Model file for the job. Use its own axes, mm. A direction names the side the tool comes from. Round coordinates to 2 decimals unless told otherwise and drop trailing zeros. Loops run counter-clockwise (first coordinate to the right, second up) from the corner with the lowest first, then second, coordinate; pieces in that order, holes last. Notation, with made-up numbers: M -4,5 L 11,5 A12 ccw 11,10 Z; hole C 28.5,-15.75 d1. An arc over 180 degrees is marked long. Answer in a Markdown table with one row per item.
Autodesk Inventor part; units mm, degrees
ref_plane "YZ Plane" through (0, 0, 0) normal (1, 0, 0) x (0, 1, 0)
ref_plane "XZ Plane" through (0, 0, 0) normal (0, 1, 0) x (-1, 0, 0)
ref_plane "XY Plane" through (0, 0, 0) normal (0, 0, 1) x (1, 0, 0)
sketch "Sketch1" plane through (0, 0, 0) normal (0, 0, 1) x (1, 0, 0)
  line L0 (0, 0) -> (-78.3, 0)
  line L1 (-78.3, 0) -> (-78.3, 100)
  line L2 (-78.3, 100) -> (0, 100)
  line L3 (0, 100) -> (0, 0)
  circle A0 centre (-11.5, 10) radius 1.5
  circle A1 centre (-11.5, 31.4) radius 1.5
  circle A2 centre (-14.5, 48.9) radius 1.5
  circle A3 centre (-27.5, 48.9) radius 1.5
  circle A4 centre (-70.8, 92.5) radius 1.5
  circle A5 centre (-70.8, 82.5) radius 1.5
  circle A6 centre (-70.8, 72.5) radius 1.5
  line L4 (0, 56.4) -> (-28.3, 56.4)
  line L5 (-28.3, 56.4) -> (-58.3, 86.4)
  line L6 (-58.3, 86.4) -> (-58.3, 100)
  line L7 (-30, 0) -> (-78.3, 48.3)
  dimension "d0" = 100
  dimension "d1" = 78.3
  dimension "d2" = 3
  dimension "d3" = 3
  dimension "d4" = 3
  dimension "d5" = 3
  dimension "d6" = 3
  dimension "d7" = 3
  dimension "d8" = 3
  dimension "d9" = 7.5
  dimension "d10" = 7.5
  dimension "d11" = 7.5
  dimension "d12" = 7.5
  dimension "d13" = 10
  dimension "d14" = 10
  dimension "d15" = 11.5
  dimension "d16" = 10
  dimension "d17" = 11.5
  dimension "d18" = 14.5
  dimension "d19" = 21.4
  dimension "d23" = 28.3
  dimension "d24" = 135
  dimension "d25" = 135
  dimension "d26" = 48.3
  dimension "d27" = 56.4
  dimension "d28" = 20
  dimension "d31" = 13
  dimension "d32" = 17.5
  dimension "d45" = 17.5
extrude "Extrusion1" add sketch "Sketch1" along normal blind 6 contours L0 L7 L1 L2 L6 L5 L4 L3
sketch "Sketch2" plane through (0, 0, 6) normal (0, 0, 1) x (1, 0, 0)
  line L0 (-30, 0) -> (0, 0)
  line L1 (0, 56.4) -> (-28.3, 56.4)
  line L2 (0, 0) -> (-4, 0)
  line L3 (-4, 0) -> (-4, 56.4)
  line L4 (-4, 56.4) -> (0, 56.4)
  line L5 (0, 56.4) -> (0, 0)
  dimension "d33" = 4
extrude "Extrusion2" cut sketch "Sketch2" against normal blind 6
sketch "Sketch3" plane through (0, 0, 6) normal (0, 0, 1) x (1, 0, 0)
  circle A0 centre (-11.5, 10) radius 1.5
  circle A1 centre (-11.5, 31.4) radius 1.5
  circle A2 centre (-11.5, 10) radius 2.75
  circle A3 centre (-11.5, 31.4) radius 1.5
  circle A4 centre (-11.5, 31.4) radius 2.75
  circle A5 centre (-14.5, 48.9) radius 1.5
  circle A6 centre (-27.5, 48.9) radius 1.5
  circle A7 centre (-70.8, 72.5) radius 1.5
  circle A8 centre (-70.8, 82.5) radius 1.5
  circle A9 centre (-70.8, 92.5) radius 1.5
  circle A10 centre (-14.5, 48.9) radius 1.5
  circle A11 centre (-14.5, 48.9) radius 2.75
  circle A12 centre (-27.5, 48.9) radius 1.5
  circle A13 centre (-27.5, 48.9) radius 2.75
  circle A14 centre (-70.8, 72.5) radius 1.5
  circle A15 centre (-70.8, 72.5) radius 2.75
  circle A16 centre (-70.8, 82.5) radius 1.5
  circle A17 centre (-70.8, 82.5) radius 2.75
  circle A18 centre (-70.8, 92.5) radius 1.5
  circle A19 centre (-70.8, 92.5) radius 2.75
  point P0 (0, 0)
  dimension "d36" = 5.5
  dimension "d37" = 5.5
  dimension "d40" = 5.5
  dimension "d41" = 5.5
  dimension "d42" = 5.5
  dimension "d43" = 5.5
  dimension "d44" = 5.5
extrude "Extrusion3" cut sketch "Sketch3" against normal blind 2 contours A0 | A1 | A2 | A4 | A5 | A6 | A7 | A8 | A9 | A11 | A13 | A15 | A17 | A19
equation "\"d10\" = d9"
equation "\"d11\" = d9"
equation "\"d12\" = d11"
equation "\"d14\" = d13"
equation "\"d17\" = d15"
equation "\"d25\" = d24"
properties part number "Plate_standard_low_3D" material "Aluminum 6061, Welded"
1. Wall check: probe 1 along X at (y, z) = (48.9, 0.9); probe 2 along Y at (x, z) = (-11.5, 1.1); probe 3 along X at (y, z) = (10, 1.7). Give the ranges that are in metal, low to high.
Verdict:
| item | result |
|---|---|
| probe 1 | x = -78.3 to -29, -26 to -16, -13 to -4 |
| probe 2 | y = 0 to 8.5, 11.5 to 29.9, 32.9 to 56.4 |
| probe 3 | x = -40 to -13, -10 to -4 |
2. Pin check, flat tips, straight feed: pin 1 (2 mm diameter, centred on x = -25, z = 4, fed in from +Y); pin 2 (1 mm diameter, centred on x = -46, z = 2, fed in from -Y); pin 3 (5 mm diameter, centred on x = -70.8, y = 72.5, fed in from +Z); pin 4 (1.8 mm diameter, centred on x = -70.8, y = 92.5, fed in from +Z). Stop position of each tip, or through.
Verdict:
| item | result |
|---|---|
| pin 1 | stops at y = 56.4 |
| pin 2 | stops at y = 15.5 |
| pin 3 | stops at z = 4 |
| pin 4 | passes through |
3. Saw through at A-A (y = 82.5). Write the cut outline in (x, z), and give its area (3 significant figures).
Verdict:
| item | result |
|---|---|
| outline | M -78.3,0 L -72.3,0 L -72.3,4 L -73.55,4 L -73.55,6 L -78.3,6 Z; M -69.3,0 L -54.4,0 L -54.4,6 L -68.05,6 L -68.05,4 L -69.3,4 Z |
| area | 120 mm² |
4. Saw through at C-C (x = -70.8). Write the cut outline in (y, z), and give its area (3 significant figures).
Verdict:
| item | result |
|---|---|
| outline | M 40.8,0 L 71,0 L 71,4 L 69.75,4 L 69.75,6 L 40.8,6 Z; M 74,0 L 81,0 L 81,4 L 79.75,4 L 79.75,6 L 75.25,6 L 75.25,4 L 74,4 Z; M 84,0 L 91,0 L 91,4 L 89.75,4 L 89.75,6 L 85.25,6 L 85.25,4 L 84,4 Z; M 94,0 L 100,0 L 100,6 L 95.25,6 L 95.25,4 L 94,4 Z |
| area | 286 mm² |
5. Tool access for faces 5 (the cylindrical face through (-69.994, 71.235, 1.972)), 6 (the cylindrical face through (-14.858, 51.627, 5.014)): list every direction of +Z, -Z, +X, -X, +Y, -Y with a clear straight run to the whole face (end or side of a thin tool).
Verdict:
| item | result |
|---|---|
| face 5 | +Z, -Z |
| face 6 | +Z |
6. Saw through at B-B (z = 2.8). Write the cut outline in (x, y).
Verdict:
| item | result |
|---|---|
| outline | M -78.3,48.3 L -30,0 L -4,0 L -4,56.4 L -28.3,56.4 L -58.3,86.4 L -58.3,100 L -78.3,100 Z; hole C -70.8,72.5 d3; hole C -70.8,82.5 d3; hole C -70.8,92.5 d3; hole C -27.5,48.9 d3; hole C -14.5,48.9 d3; hole C -11.5,10 d3; hole C -11.5,31.4 d3 |
7. Mould opens along Y. For faces 1 (the flat face through (-70, 81, 4)), 2 (the flat face through (-68, 100, 3)), 3 (the cylindrical face through (-72.827, 74.359, 5.014)), 4 (the flat face through (-42, 51, 6)) say: +Y half, -Y half, draft (parallel to the pull), parting line (faces both ways), or undercut.
Verdict:
| item | result |
|---|---|
| face 1 | undercut |
| face 2 | +Y half |
| face 3 | undercut |
| face 4 | draft |
8. Saw through at D-D (y = 72.5). Write the cut outline in (x, z).
Verdict:
| item | result |
|---|---|
| outline | M -78.3,0 L -72.3,0 L -72.3,4 L -73.55,4 L -73.55,6 L -78.3,6 Z; M -69.3,0 L -44.4,0 L -44.4,6 L -68.05,6 L -68.05,4 L -69.3,4 Z |
